from build123d import *

# Parameters (mm, degrees)
F0_R     = 89.73439
F0_R_2   = 3.175
F0_R_3   = 26.9875
F1_DEPTH = 20.6375
F2_DEPTH = 7.9375
F3_R     = 6.35
F3_R_2   = 3.175
F4_DEPTH = 5.08
F5_SIZE  = 1.524
F6_SIZE  = 0.381


with BuildPart() as f1:
    # F0 (on Front) → F1 (new body)
    with BuildSketch(Plane.XZ):
        Circle(F0_R)
        with Locations((0, -70.74916)):
            Circle(F0_R_2, mode=Mode.SUBTRACT)
        with Locations((-70.74916, 0)):
            Circle(F0_R_2, mode=Mode.SUBTRACT)
        Circle(F0_R_3, mode=Mode.SUBTRACT)
        with Locations((70.74916, 0)):
            Circle(F0_R_2, mode=Mode.SUBTRACT)
        with Locations((0, 70.74916)):
            Circle(F0_R_2, mode=Mode.SUBTRACT)
        Circle(F0_R_3)
        with BuildLine():
            ThreePointArc((4.7625, 20.080463), (0, -20.6375), (-4.7625, 20.080463))
            Line((-4.7625, 20.080463), (-4.7625, 25.4))
            Line((-4.7625, 25.4), (4.7625, 25.4))
            Line((4.7625, 25.4), (4.7625, 20.080463))
        make_face(mode=Mode.SUBTRACT)
    extrude(amount=F1_DEPTH)

    # F0 (on Front) → F2 (cut)
    with BuildSketch(Plane.XZ):
        Circle(F0_R_3)
        with BuildLine():
            ThreePointArc((4.7625, 20.080463), (0, -20.6375), (-4.7625, 20.080463))
            Line((-4.7625, 20.080463), (-4.7625, 25.4))
            Line((-4.7625, 25.4), (4.7625, 25.4))
            Line((4.7625, 25.4), (4.7625, 20.080463))
        make_face(mode=Mode.SUBTRACT)
    extrude(amount=F2_DEPTH, mode=Mode.SUBTRACT)

    # F3 (on face) → F4 (cut)
    with BuildSketch(Plane.XZ.offset(20.6375)):
        with Locations((0, 70.74916)):
            Circle(F3_R)
        with Locations((0, 70.74916)):
            Circle(F3_R_2, mode=Mode.SUBTRACT)
        with Locations((-70.74916, 0)):
            Circle(F3_R)
        with Locations((-70.74916, 0)):
            Circle(F3_R_2, mode=Mode.SUBTRACT)
        with Locations((0, -70.74916)):
            Circle(F3_R)
        with Locations((0, -70.74916)):
            Circle(F3_R_2, mode=Mode.SUBTRACT)
        with Locations((70.74916, 0)):
            Circle(F3_R)
        with Locations((70.74916, 0)):
            Circle(F3_R_2, mode=Mode.SUBTRACT)
    extrude(amount=-F4_DEPTH, mode=Mode.SUBTRACT)

    # F5
    f5_edges = [f1.edges().sort_by_distance(p)[0] for p in [
        (89.73439, -10.31875, 0),
        (-89.73439, 0, 0),
        (-89.73439, -20.6375, 0),
    ]]
    chamfer(f5_edges, length=F5_SIZE)

    # F6
    f6_edges = [f1.edges().sort_by_distance(p)[0] for p in [
        (0, -20.6375, -20.6375),
        (-77.09916, -20.6375, 0),
        (-6.35, -20.6375, 70.74916),
        (64.39916, -20.6375, 0),
        (-6.35, -20.6375, -70.74916),
        (0, -7.9375, -20.6375),
    ]]
    chamfer(f6_edges, length=F6_SIZE)


solid = f1.part
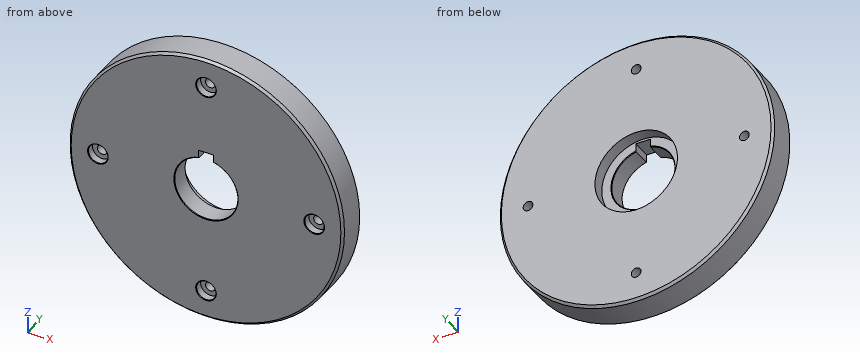
Geometry check sheet. Reference: the model listing, model coordinates, mm. Round coordinates to 2 decimals unless told otherwise and drop trailing zeros.
Item 1: Gauge pin test, flat ends, axial feed: pin 1 (14 mm diameter, centred on x = 72.5, z = -2.5, fed in from -Y); pin 2 (3 mm diameter, centred on x = -51, y = -8, fed in from -Z); pin 3 (4.5 mm diameter, centred on y = -16.5, z = 21.5, fed in from -X); pin 4 (1.5 mm diameter, centred on x = -4.5, y = -5, fed in from +Z). Record the tip position at first contact, or that the pin passes through.
Item 2: Cross-section at A-A on x = 0. Count the separate pieces of the cut face and the enclosed holes in it, then the cut area to 3 significant figures.
Item 3: Thickness scan on line 1 (Z direction, x = 0, y = -17.55); line 2 (Z direction, x = 0, y = -7.5); line 3 (X direction, y = -2, z = 7). Record the ranges inside material, lowest first.
Answer sheet:
1. pin 1: stops at y = -20.64
1. pin 2: stops at z = -74.85
1. pin 3: stops at x = -87.65
1. pin 4: stops at z = 89.66
2. separate pieces: 4
2. enclosed holes: 0
2. area: 2,360 mm2
3. line 1: z = -89.73 to -77.1, -64.4 to -20.64, 25.4 to 64.4, 77.1 to 89.73
3. line 2: z = -89.73 to -73.92, -67.57 to -26.99, 26.99 to 67.57, 73.92 to 89.73
3. line 3: x = -89.46 to -26.06, 26.06 to 89.46
